Check sheet for the modelled part. Datum: model origin and axes. Units: mm. Face numbers are marked on the shaded views. A direction names the side the tool comes from. Give positions to 0.01 mm unless a question says otherwise; leave off trailing zeros. Write each loop counter-clockwise with the first axis right and the second up, starting at its lowest first coordinate (ties: lowest second). Pieces come first, ordered by that corner, then holes. Notation, with made-up numbers: M 56.5,14 L 90.5,14 A20 cw 90.5,43 Z; hole C 73.5,47.5 d8. An arc over 180 degrees is marked long. Use CSV: the item, a comma, the result in double quotes. Start each with the question number.
1. Cross-section at C-C, the plane x = -4. Enter the section's corners in (y, z), and give its area (3 significant figures).
2. Depth check by flat-ended pin: P1, Ø8.5, axis at y = 10.5, z = -3.5, coming from the -X side; P2, Ø12, axis at x = -30, z = -2.5, coming from the +Y side; P3, Ø2, axis at x = 2, y = 35.5, coming from the +Z side. Enter the tip coordinate at first touch or a pass-through.
3. Cross-section at B-B, the plane y = 16. Enter the section's corners in (x, z), and give its area (3 significant figures).
4. Scan lines: line 1 (Z direction, x = -4.5, y = 7.5); line 2 (X direction, y = 3, z = 2); line 3 (Z direction, x = -21, y = 33). Record each from-to range of solid material in increasing order.
5. Cross-section at D-D, the plane x = 29. Enter the section's corners in (y, z), and give its area (3 significant figures).
6. Cross-section at A-A, the plane z = 0. Enter the section's corners in (x, y), and give its area (3 significant figures).
7. Access from +Z, -Z, +X, -X, +Y, -Y to the whole of each face (thin tool, end or side, straight path). Record for the marked faces 1, 2 and 3.
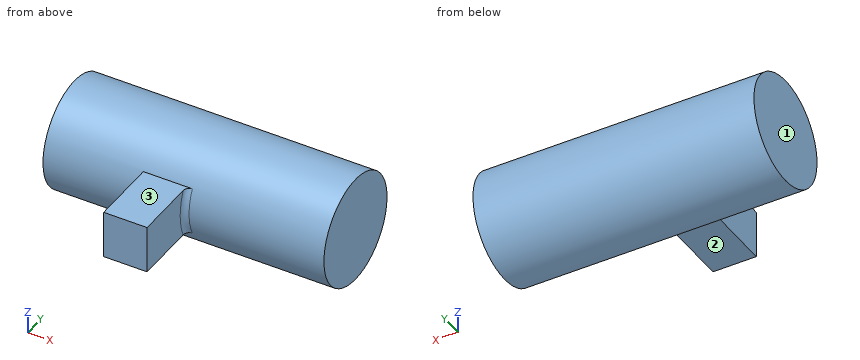
from build123d import *

# Parameters (mm, degrees)
SKETCH_1_W           = 15.445067976
SKETCH_1_H           = 17.0246772
EXTRUDE_1_DEPTH      = 50
EXTRUDE_2_DEPTH      = 50
EXTRUDE_2_DEPTH_BACK = 50
SKETCH_2_R           = 19.191040977
FILLET_3_R           = 2


with BuildPart() as part:
    # 草图1 → 凸台-拉伸1 (new body)
    with BuildSketch(Plane(origin=(0, 0, 0), x_dir=(1, 0, 0), z_dir=(0, 1, 0))):
        Rectangle(SKETCH_1_W, SKETCH_1_H)
    extrude(amount=EXTRUDE_1_DEPTH)

    # 草图2 → 凸台-拉伸2 (add, two sides: drawn at the far end of the back side and taken through both)
    with BuildSketch(Plane(origin=(7.722533988, 0, 0), x_dir=(0, 0, -1), z_dir=(1, 0, 0)).offset(-EXTRUDE_2_DEPTH_BACK)):
        with Locations((0, 41.312136517)):
            Circle(SKETCH_2_R)
    extrude(amount=EXTRUDE_2_DEPTH + EXTRUDE_2_DEPTH_BACK)

    # 圆角3
    # the kernel refuses this fillet: 2 mm, written as the material it adds along each edge
    with BuildSketch(Plane(origin=(7.722533988, 41.312136517, 0), x_dir=(0, -0.7517142761643256, 0.6594889286491047), z_dir=(0, 0.6594889286491047, 0.7517142761643256))) as fillet_3_piece_1_section:
        with BuildLine():
            CenterArc((19.191040977 + FILLET_3_R, FILLET_3_R), FILLET_3_R, 180, 90)
            Line((19.191040977, FILLET_3_R), (19.191040977, 0))
            Line((19.191040977, 0), (19.191040977 + FILLET_3_R, 0))
        make_face()
    fillet_3_piece_1 = revolve(axis=Axis((7.722533988, 41.312136517, 0), (1, 0, 0)), revolution_arc=82.521814453, mode=Mode.PRIVATE)
    fillet_3_piece_1 = split(fillet_3_piece_1, bisect_by=Plane(origin=(8.28980216, 21.553827368, -8.5123386), z_dir=(0, 0, 1)), keep=Keep.TOP, mode=Mode.PRIVATE)
    fillet_3_piece_1 = split(fillet_3_piece_1, bisect_by=Plane(origin=(8.28980216, 21.553827368, 8.5123386), z_dir=(0, 0, -1)), keep=Keep.TOP, mode=Mode.PRIVATE)
    add(fillet_3_piece_1)


solid = part.part
Worked answers:
1,outline,"M 0,-8.51 L 24.11,-8.51 A19.19 ccw long 24.11,8.51 L 0,8.51 Z"
1,area,"1,540 mm^2"
2,P1,"stops at x = -7.72"
2,P2,"stops at y = 60.5"
2,P3,"stops at z = 18.58"
3,outline,"M -7.72,-8.51 L 7.72,-8.51 L 7.72,8.51 L -7.72,8.51 Z"
3,area,"263 mm^2"
4,line 1,"z = -8.51 to 8.51"
4,line 2,"x = -7.72 to 7.72"
4,line 3,"z = -17.3 to 17.3"
5,outline,"C 41.31,0 d38.38"
5,area,"1,160 mm^2"
6,outline,"M -42.28,22.12 L -7.72,22.12 L -7.72,0 L 7.72,0 L 7.72,20.12 A2 cw 9.72,22.12 L 57.72,22.12 L 57.72,60.5 L -42.28,60.5 Z"
6,area,"4,180 mm^2"
7,face 1,"+Z, -Z, -X, +Y, -Y"
7,face 2,"-Z, +X, -X, -Y"
7,face 3,"+Z, +X, -X, -Y"
